```python
from build123d import *

# Parameters (mm, degrees)
F1_DEPTH = 20
F3_D     = 5.2
F3_DEPTH = 10
F3_TIP   = 1.5622376095


with BuildPart() as f1:
    # F0 (on Front) → F1 (new body)
    with BuildSketch(Plane.XZ):
        Polygon((0, -65), (0, 0), (-48, 0), (-48, -10), (-33, -10), (-15, -65), align=None)
    extrude(amount=F1_DEPTH)

    # F3
    with Locations(Plane.YZ):
        with Locations((-10, -27.3), (-10, -57.3)):
            Hole(F3_D / 2, depth=F3_DEPTH)
            with Locations((0, 0, -(F3_DEPTH + F3_TIP / 2))):  # 118° drill point
                Cone(0, F3_D / 2, F3_TIP, mode=Mode.SUBTRACT)


solid = f1.part
```
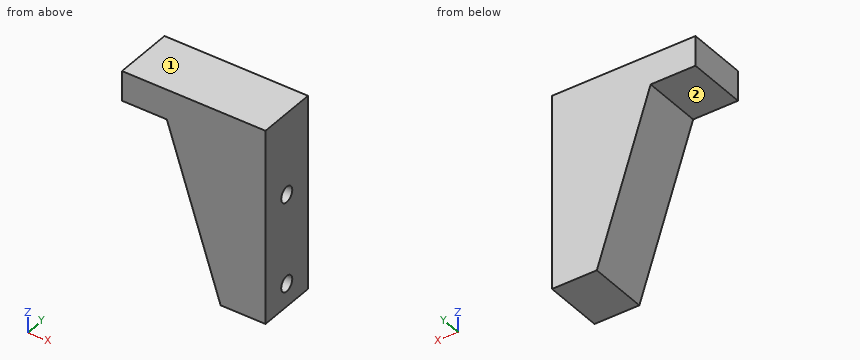
Geometry check sheet. Reference: the model listing, model coordinates, mm. Face numbers are marked on the shaded views. A direction names the side the tool comes from. Round coordinates to 2 decimals unless told otherwise and drop trailing zeros. Order: outer loops, then holes, each group sorted by start corner. A loop starts at its lowest first (then second) coordinate and runs counter-clockwise, first axis right, second up. Notation, with made-up numbers: (71, 49.5) -> (76, 49.5) arc R22 ccw to (76, 55.5) -> close; hole circle Ø1 at (47.25, 12). An arc over 180 degrees is marked (long way). Return JSON: item names as keys, results as strings. Group by question number.
Q1. Material ranges on probe 1 along Z at (x, y) = (-6.25, -10); probe 2 along Y at (x, z) = (-6.5, -57.3); probe 3 along Z at (x, y) = (-3.5, -8.25), recorded low to high. Write a range as from..to.
Q2. Gauge pin test, flat ends, axial feed: pin 1 (4.5 mm diameter, centred on y = -10, z = -57.3, fed in from -X); pin 2 (8 mm diameter, centred on x = -26, z = -49.5, fed in from +Y); pin 3 (6 mm diameter, centred on y = -10, z = -27.3, fed in from -X); pin 4 (6 mm diameter, centred on y = -15.5, z = -37, fed in from -X). Record the tip position at first contact, or that the pin passes through.
Q3. Section check A-A, the plane y = -5.5. Record the boundary of the cut face in (x, z), plus the area to 3 significant figures.
Q4. Section check C-C, the plane x = -24.5. Record the boundary of the cut face in (y, z).
Q5. Tool access check on the marked faces 1 and 2. Record the directions out of +Z, -Z, +X, -X, +Y, -Y that give a thin tool (end or side, any length) a straight path to the whole face; none if there is none.
Q6. Section check B-B, the plane z = -35.5. Record the boundary of the cut face in (x, y).
Numbers:
{
 "1": {"probe 1": "-65..-59.9, -54.7..-29.9, -24.7..0", "probe 2": "-20..-12.6, -7.4..0", "probe 3": "-65..-59.22, -55.38..-29.22, -25.38..0"},
 "2": {"pin 1": "x = -18.26", "pin 2": "through", "pin 3": "x = -28.32", "pin 4": "x = -25.15"},
 "3": {"outline": "(-48, -10) -> (-33, -10) -> (-15, -65) -> (0, -65) -> (0, 0) -> (-48, 0) -> close", "area": "1,800 mm^2"},
 "4": {"outline": "(-20, -35.97) -> (0, -35.97) -> (0, 0) -> (-20, 0) -> close"},
 "5": {"face 1": "+Z, +X, -X, +Y, -Y", "face 2": "-Z, -X, +Y, -Y"},
 "6": {"outline": "(-24.65, -20) -> (0, -20) -> (0, 0) -> (-24.65, 0) -> close"}
}
